from build123d import *

# Parameters (mm, degrees)
MIEMBRO_ESTRUCTURAL1_DEPTH        = 1412
TALADRO_DE_MARGEN_PARA_M161_D     = 17.5
TALADRO_DE_MARGEN_PARA_M161_DEPTH = 2.5


with BuildPart() as part:
    # Sketch1 → Miembro estructural1 (new body)
    with BuildSketch(Plane.YZ.offset(-623.635182539)):
        with BuildLine():
            Line((-12.3, -25), (12.3, -25))
            ThreePointArc((12.3, -25), (21.280256121, -21.280256121), (25, -12.3))
            Line((25, -12.3), (25, 12.3))
            ThreePointArc((25, 12.3), (21.280256121, 21.280256121), (12.3, 25))
            Line((12.3, 25), (-12.3, 25))
            ThreePointArc((-12.3, 25), (-21.280256121, 21.280256121), (-25, 12.3))
            Line((-25, 12.3), (-25, -12.3))
            ThreePointArc((-25, -12.3), (-21.280256121, -21.280256121), (-12.3, -25))
        make_face()
        with BuildLine():
            Line((-12.3, -22.5), (12.3, -22.5))
            ThreePointArc((12.3, -22.5), (19.512489168, -19.512489168), (22.5, -12.3))
            Line((22.5, -12.3), (22.5, 12.3))
            ThreePointArc((22.5, 12.3), (19.512489168, 19.512489168), (12.3, 22.5))
            Line((12.3, 22.5), (-12.3, 22.5))
            ThreePointArc((-12.3, 22.5), (-19.512489168, 19.512489168), (-22.5, 12.3))
            Line((-22.5, 12.3), (-22.5, -12.3))
            ThreePointArc((-22.5, -12.3), (-19.512489168, -19.512489168), (-12.3, -22.5))
        make_face(mode=Mode.SUBTRACT)
    extrude(amount=MIEMBRO_ESTRUCTURAL1_DEPTH)

    # Taladro de margen para M161
    with Locations(Plane(origin=(0, -25, 0), x_dir=(-1, 0, 0), z_dir=(0, -1, 0))):
        with Locations((-152.364817461, 0), (-212.364817461, 0)):
            Hole(TALADRO_DE_MARGEN_PARA_M161_D / 2, depth=TALADRO_DE_MARGEN_PARA_M161_DEPTH)


solid = part.part
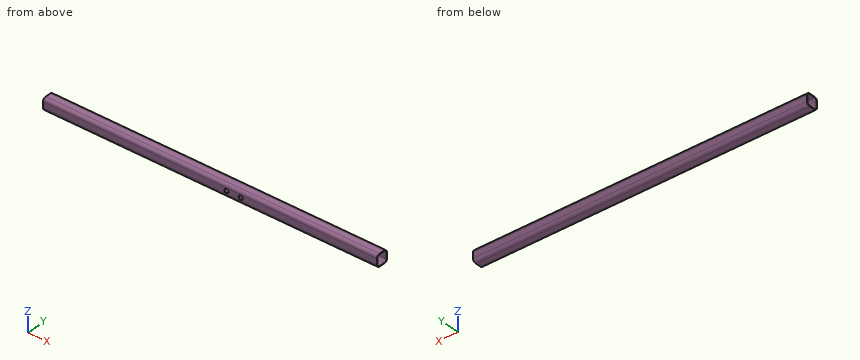
CAD build for the part. Positions are in the model's coordinates, mm. Give positions to 0.01 mm unless a question says otherwise; leave off trailing zeros. Order: outer loops, then holes, each group sorted by start corner. A loop starts at its lowest first (then second) coordinate and runs counter-clockwise, first axis right, second up. Notation, with made-up numbers: (-26, -8) -> (-9, -8) arc R27 ccw to (-9, 13) -> close; hole circle Ø3 at (81.25, 39.5). An arc over 180 degrees is marked (long way). Return JSON: item names as keys, results as strings.
Q1. Saw through at A-A (y = 0). Write the cut outline in (x, z).
Working result:
{"outline": "(-623.64, -25) -> (788.36, -25) -> (788.36, -22.5) -> (-623.64, -22.5) -> close; (-623.64, 22.5) -> (788.36, 22.5) -> (788.36, 25) -> (-623.64, 25) -> close"}
Q2. Saw through at C-C (z = 0). Write the cut outline in (x, y), then the cut area to 3 significant figures.
Working result:
{"outline": "(-623.64, -25) -> (143.61, -25) -> (143.61, -22.5) -> (-623.64, -22.5) -> close; (-623.64, 22.5) -> (788.36, 22.5) -> (788.36, 25) -> (-623.64, 25) -> close; (161.11, -25) -> (203.61, -25) -> (203.61, -22.5) -> (161.11, -22.5) -> close; (221.11, -25) -> (788.36, -25) -> (788.36, -22.5) -> (221.11, -22.5) -> close", "area": "6,970 mm²"}
Q3. Flat gauge pins, fed straight in: pin 1 (16 mm diameter, centred on x = 152.36, z = 0, fed in from -Y); pin 2 (8 mm diameter, centred on x = -171, y = -18.5, fed in from -Z). Where does each tip first touch, or does it go through?
Working result:
{"pin 1": "y = 22.5", "pin 2": "z = -24.81"}
Q4. Drill centre lines: line 1 (Z direction, x = -497.5, y = -7); line 2 (Y direction, x = 219.5, z = 14). Where is each one in solid material? Low to high.
Working result:
{"line 1": "-25 to -22.5, 22.5 to 25", "line 2": "-24.89 to -22.36, 22.36 to 24.89"}
Q5. Saw through at B-B (x = 627). Write the cut outline in (y, z), then the cut area to 3 significant figures.
Working result:
{"outline": "(-25, -12.3) arc R12.7 ccw to (-12.3, -25) -> (12.3, -25) arc R12.7 ccw to (25, -12.3) -> (25, 12.3) arc R12.7 ccw to (12.3, 25) -> (-12.3, 25) arc R12.7 ccw to (-25, 12.3) -> close; hole (-22.5, -12.3) arc R10.2 ccw to (-12.3, -22.5) -> (12.3, -22.5) arc R10.2 ccw to (22.5, -12.3) -> (22.5, 12.3) arc R10.2 ccw to (12.3, 22.5) -> (-12.3, 22.5) arc R10.2 ccw to (-22.5, 12.3) -> close", "area": "426 mm²"}
